```python
from build123d import *

# Parameters (mm, degrees)
BOSS_EXTRUDE1_DEPTH = 15
CUT_EXTRUDE1_DEPTH  = 10
FILLET1_R           = 10


with BuildPart() as part:
    # Sketch2 → Boss-Extrude1 (new body)
    with BuildSketch(Plane.XY):
        with BuildLine():
            Line((-40, -144.568322948), (-40, -64.568322948))
            Line((-40, -64.568322948), (40, -64.568322948))
            Line((40, -64.568322948), (40, -144.568322948))
            ThreePointArc((40, -144.568322948), (0, -150), (-40, -144.568322948))
        make_face()
    extrude(amount=BOSS_EXTRUDE1_DEPTH)

    # Sketch3 → Cut-Extrude1 (cut)
    with BuildSketch(Plane.XY.offset(15)):
        with BuildLine():
            Line((-40, -137.291660344), (-40, -64.568322948))
            Line((-40, -64.568322948), (40, -64.568322948))
            Line((40, -64.568322948), (40, -137.291660344))
            ThreePointArc((40, -137.291660344), (0, -143), (-40, -137.291660344))
        make_face()
    extrude(amount=-CUT_EXTRUDE1_DEPTH, mode=Mode.SUBTRACT)

    # Fillet1
    fillet1_edges = [part.edges().sort_by_distance(p)[0] for p in [
        (0, -150, 0),
    ]]
    fillet(fillet1_edges, radius=FILLET1_R)


solid = part.part
```
Source: CAD feature listing. Evaluate the final solid. Frame: model axes, mm. Round coordinates to 2 decimals unless told otherwise and drop trailing zeros. Loops run counter-clockwise (first coordinate to the right, second up) from the corner with the lowest first, then second, coordinate; pieces in that order, holes last. Notation, with made-up numbers: M 76,-16.75 L 89,-16.75 A8 ccw 89,-9.75 Z; hole C 60.25,22 d11. An arc over 180 degrees is marked long. Use a Markdown table: item, result. Add a question column.
1. Cut plane A-A, the plane y = -119.5. Output: boundary loops of the cut face in (x, z).
2. Cut plane B-B, the plane z = 1.5. Output: boundary loops of the cut face in (x, y).
3. Ray query, line 1 along Z through (x, y) = (0.5, -88); line 2 along Y through (x, z) = (7.5, 7.5); line 3 along Y through (x, z) = (5, 7.25). Return the intervals inside material, ascending. Write a range as [from, to].
4. Contact query for flat-ended pins moving along their axis: pin 1 (4 mm diameter, centred on x = -22.5, z = 11, fed in from -Y); pin 2 (1.5 mm diameter, centred on x = -27, z = 9.5, fed in from +Y). Output: stop coordinate, or through.
5. Pull-direction query (X, two-part tool) for faces 1 (the cylindrical face through (0.6, -150, 12.5)), 2 (the flat face through (1, -102, 0)), 3 (the flat face through (-40, -114, 4)), 4 (the cylindrical face through (0.6, -143, 10.1)); classes: +X half, -X half, draft (parallel to the pull), parting line (faces both ways), or undercut.
Solution:
| question | item | result |
|---|---|---|
| 1 | outline | M -40,0 L 40,0 L 40,5 L -40,5 Z |
| 2 | outline | M -40,-139.65 A145.27 ccw 40,-139.65 L 40,-64.57 L -40,-64.57 Z |
| 3 | line 1 | z = [0, 5] |
| 3 | line 2 | y = [-149.49, -142.8] |
| 3 | line 3 | y = [-149.53, -142.91] |
| 4 | pin 1 | stops at y = -148.59 |
| 4 | pin 2 | stops at y = -140.28 |
| 5 | face 1 | parting line |
| 5 | face 2 | draft |
| 5 | face 3 | -X half |
| 5 | face 4 | undercut |
